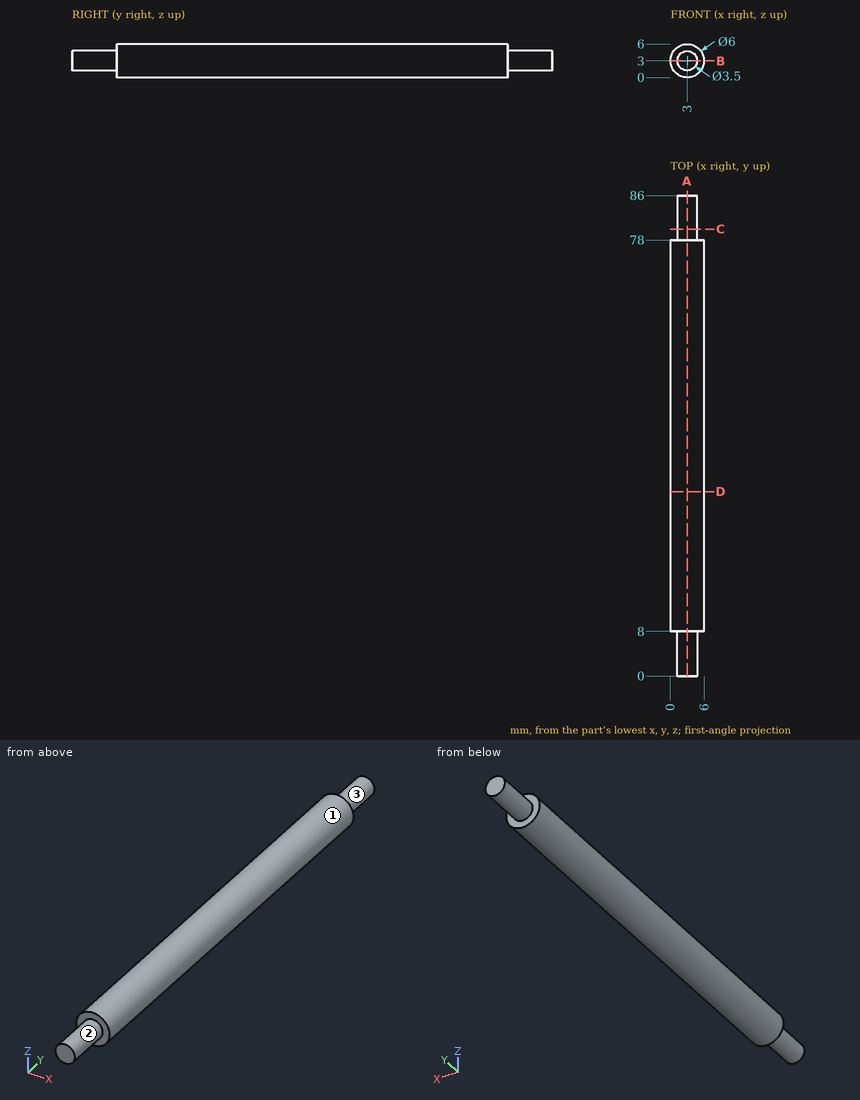
Design review of the part shown in the three views and the two pictorial views. Dimensions are in mm from the part's minimum x, y and z. A direction names the side the tool comes from. Coordinates: 2 decimals unless noted, no trailing zeros. Loops run counter-clockwise (first coordinate to the right, second up) from the corner with the lowest first, then second, coordinate; pieces in that order, holes last. Notation, with made-up numbers: M 56,84 L 70,84 A26 cw 70,107 Z; hole C -18.5,-14.5 d9. An arc over 180 degrees is marked long. Put each result on its own line as item: value. Start each with the question number.
Q1. Add section A-A (x = 3). Write out the cut boundary in (y, z), and give its area (3 significant figures).
Q2. Clearance check with a flat-ended pin moving along its axis: pin 1 (2 mm diameter, centred on x = 1, y = 55.5, fed in from -Z). State where the tip first meets the part, or that it passes through.
Q3. Add section B-B (z = 3). Write out the cut boundary in (x, y).
Q4. For the marked faces 1, 2 and 3, list the 3-axis set-ups (+Z, -Z, +X, -X, +Y, -Y) from which the entire face can be reached by the end or side of a thin tool; tool diameter is ignored.
Q5. Add section D-D (y = 33). Write out the cut boundary in (x, z), and give its area (3 significant figures).
Q6. Wall thickness on line 1 (Y direction, x = 4.6, z = 2.15); line 2 (Z direction, x = 3.25, y = 50): over which ranges is each line inside the solid? List them lowest first.
Q7. Add section C-C (y = 80). Write out the cut boundary in (x, z).
Answers:
1. outline: M 0,1.25 L 8,1.25 L 8,0 L 78,0 L 78,1.25 L 86,1.25 L 86,4.75 L 78,4.75 L 78,6 L 8,6 L 8,4.75 L 0,4.75 Z
1. area: 476 mm^2
2. pin 1: stops at z = 0.17
3. outline: M 0,8 L 1.25,8 L 1.25,0 L 4.75,0 L 4.75,8 L 6,8 L 6,78 L 4.75,78 L 4.75,86 L 1.25,86 L 1.25,78 L 0,78 Z
4. face 1: +Y, -Y
4. face 2: -Y
4. face 3: +Y
5. outline: C 3,3 d6
5. area: 28.3 mm^2
6. line 1: y = 8 to 78
6. line 2: z = 0.01 to 5.99
7. outline: C 3,3 d3.5
